Could you check a few things on this model? Use its own coordinates, in mm. A direction names the side the tool comes from. Round coordinates to 2 decimals unless told otherwise and drop trailing zeros. Loops run counter-clockwise (first coordinate to the right, second up) from the corner with the lowest first, then second, coordinate; pieces in that order, holes last. Notation, with made-up numbers: (13, 33) -> (29, 33) arc R27 ccw to (29, 65) -> close; hole circle Ø7 at (63.5, 42). An arc over 180 degrees is marked (long way). Put each result on its own line as item: value. Start each with the question number.
1. Imagine slicing it at B-B, the plane y = -260. Please give me the cut outline in (x, z), and give its area (3 significant figures).
2. Imagine slicing it at C-C, the plane z = -105.5. Please give me the cut outline in (x, y), and give its area (3 significant figures).
3. Which directions (+Z, -Z, +X, -X, +Y, -Y) give clear straight access to the entire face, cutting with the end or side of a thin tool? Please do faces 1 (the flat face through (-6, -1099, -199.219)), 2 (the flat face through (0, -1249, 296.516)), 3 (the flat face through (-350.63, -1099, 72)).
4. Imagine slicing it at D-D, the plane z = 378. Please give me the cut outline in (x, y).
5. Imagine slicing it at A-A, the plane x = 279. Please give me the cut outline in (y, z).
6. I need wall thicknesses on line 1 (Y direction, x = -218.5, z = 590); line 2 (Y direction, x = 207, z = 45.5); line 3 (X direction, y = -1156.5, z = 76). Which ranges of each line are inside material? Lowest first, please. Write a range as [from, to].
7. I'm going to push flat-ended pins straight in: P1, Ø10, axis at y = -473, z = 533, coming from the +X side; P2, Ø10, axis at x = 88, z = 360, coming from the -Y side; P3, Ø2, axis at x = 72, y = -1125, coming from the -Z side. Where does each tip first touch, or does it pass through?
```python
from build123d import *

# Parameters (mm, degrees)
F0_W     = 1000
F0_H     = 1000
F1_DEPTH = 1000
F2_SIZE  = 200
F3_W     = 700
F3_H     = 549.8493
F4_DEPTH = 200
F5_W     = 66.719718
F5_H     = 63.54259
F6_DEPTH = 100


with BuildPart() as f1:
    # F0 (on Front) → F1 (new body)
    with BuildSketch(Plane.XZ):
        with Locations((-0.63042, 175.785489)):
            Rectangle(F0_W, F0_H)
    extrude(amount=F1_DEPTH)

    # F2
    f2_edges = [f1.edges().sort_by_distance(p)[0] for p in [
        (-500.63042, -500, 675.785489),
        (499.36958, -500, 675.785489),
    ]]
    chamfer(f2_edges, length=F2_SIZE)

    # F3 (on face) → F4 (join)
    with BuildSketch(Plane.XZ.offset(1000)):
        with Locations((-0.63042, 75.705871)):
            Rectangle(F3_W, F3_H)
    extrude(amount=F4_DEPTH)

    # F5 (on face) → F6 (join)
    with BuildSketch(Plane.XZ.offset(1200)):
        with Locations((0.958163, 264.745094)):
            Rectangle(F5_W, F5_H)
    extrude(amount=F6_DEPTH)


solid = f1.part
```
Entries:
1. outline: (-500.63, -324.21) -> (499.37, -324.21) -> (499.37, 475.79) -> (299.37, 675.79) -> (-300.63, 675.79) -> (-500.63, 475.79) -> close
1. area: 960,000 mm^2
2. outline: (-500.63, -1000) -> (-350.63, -1000) -> (-350.63, -1200) -> (349.37, -1200) -> (349.37, -1000) -> (499.37, -1000) -> (499.37, 0) -> (-500.63, 0) -> close
2. area: 1,140,000 mm^2
3. face 1: -Z, +X, -X, -Y
3. face 2: +Z, +X, -X, -Y
3. face 3: +Z, -Z, -X, -Y
4. outline: (-500.63, -1000) -> (499.37, -1000) -> (499.37, 0) -> (-500.63, 0) -> close
5. outline: (-1200, -199.22) -> (-1000, -199.22) -> (-1000, -324.21) -> (0, -324.21) -> (0, 675.79) -> (-1000, 675.79) -> (-1000, 350.63) -> (-1200, 350.63) -> close
6. line 1: [-1000, 0]
6. line 2: [-1200, 0]
6. line 3: [-350.63, 349.37]
7. P1: x = 447.16
7. P2: y = -1000
7. P3: z = -199.22
